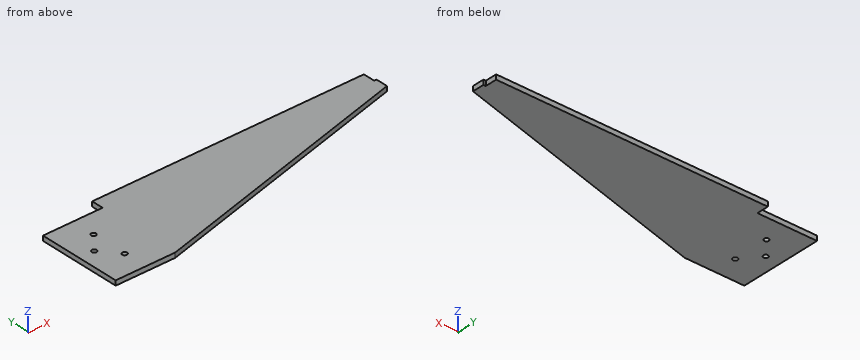
```python
from build123d import *

# Parameters (mm, degrees)
BOSS_EXTRUDE1_DEPTH = 4
BOSS_EXTRUDE2_DEPTH = 4
CUT_EXTRUDE1_REACH  = 6
SKETCH3_R           = 2


with BuildPart() as part:
    # Sketch1 → Boss-Extrude1 (new body)
    with BuildSketch(Plane.XY):
        Polygon((128, 30.092990436), (128, 40.092990436), (-100, 40.092990436), (-100, 20.092990436), (-130, 20.092990436), (-130, -39.907009564), (-100, -39.907009564), (130, 20.092990436), (130, 30.092990436), align=None)
    extrude(amount=BOSS_EXTRUDE1_DEPTH)

    # Sketch2 → Boss-Extrude2 (add)
    with BuildSketch(Plane.XY.offset(4)):
        Polygon((-100, 30.092990436), (-150, 30.092990436), (-150, -39.907009564), (-130, -39.907009564), (-130, 20.092990436), (-100, 20.092990436), align=None)
    extrude(amount=-BOSS_EXTRUDE2_DEPTH)

    # Sketch3 → Cut-Extrude1 (cut, up to next)
    with BuildSketch(Plane.XY.offset(4), mode=Mode.PRIVATE) as cut_extrude1_sk1:
        with Locations((-125, 10.092990436)):
            Circle(SKETCH3_R)
    cut_extrude1_tool1 = extrude(cut_extrude1_sk1.sketch, amount=-CUT_EXTRUDE1_REACH, mode=Mode.PRIVATE) & part.part
    add(cut_extrude1_tool1.solids().sort_by_distance((-125, 10.09299, 4))[0], mode=Mode.SUBTRACT)
    # Sketch3 → Cut-Extrude1 (cut, up to next)
    with BuildSketch(Plane.XY.offset(4), mode=Mode.PRIVATE) as cut_extrude1_sk2:
        with Locations((-125, -19.907009564)):
            Circle(SKETCH3_R)
    cut_extrude1_tool2 = extrude(cut_extrude1_sk2.sketch, amount=-CUT_EXTRUDE1_REACH, mode=Mode.PRIVATE) & part.part
    add(cut_extrude1_tool2.solids().sort_by_distance((-125, -19.90701, 4))[0], mode=Mode.SUBTRACT)
    # Sketch3 → Cut-Extrude1 (cut, up to next)
    with BuildSketch(Plane.XY.offset(4), mode=Mode.PRIVATE) as cut_extrude1_sk3:
        with Locations((-137.5, -4.907009564)):
            Circle(SKETCH3_R)
    cut_extrude1_tool3 = extrude(cut_extrude1_sk3.sketch, amount=-CUT_EXTRUDE1_REACH, mode=Mode.PRIVATE) & part.part
    add(cut_extrude1_tool3.solids().sort_by_distance((-137.5, -4.90701, 4))[0], mode=Mode.SUBTRACT)


solid = part.part
```
Geometry: final body of the model. Coordinates: model frame, mm. Give positions to 0.01 mm unless a question says otherwise; leave off trailing zeros. Write each loop counter-clockwise with the first axis right and the second up, starting at its lowest first coordinate (ties: lowest second). Pieces come first, ordered by that corner, then holes.
1. Section query B-B, the plane x = -57.5. Return loops of the section in (y, z).
2. Section query C-C, the plane y = -35. Return loops of the section in (x, z), then the cut area to 3 significant figures.
3. Pin query (flat end, axial travel): P1, Ø1.6, axis at x = 129, z = 2, coming from the +Y side; P2, Ø2, axis at x = 58, z = 2, coming from the -Y side; P3, Ø1, axis at x = 40.5, z = 0.5, coming from the -Y side. Return the tip coordinate at first contact, or that it passes through.
4. Section query A-A, the plane z = 2.95. Return loops of the section in (x, y), then the cut area to 3 significant figures.
5. Line query: probe 1 along Y at (x, z) = (-125, 1.15); probe 2 along Y at (x, z) = (-137.5, 2.6); probe 3 along X at (y, z) = (32, 2.35). Output: solid intervals per line, ascending.
Computed:
1. outline: (-28.82, 0) - (40.09, 0) - (40.09, 4) - (-28.82, 4) - close
2. outline: (-150, 0) - (-81.19, 0) - (-81.19, 4) - (-150, 4) - close
2. area: 275 mm2
3. P1: stops at y = 30.09
3. P2: stops at y = 1.05
3. P3: stops at y = -3.39
4. outline: (-150, -39.91) - (-100, -39.91) - (130, 20.09) - (130, 30.09) - (128, 30.09) - (128, 40.09) - (-100, 40.09) - (-100, 30.09) - (-150, 30.09) - close; hole circle Ø4 at (-137.5, -4.91); hole circle Ø4 at (-125, -19.91); hole circle Ø4 at (-125, 10.09)
4. area: 14,900 mm2
5. probe 1: y = -39.91 to -21.91, -17.91 to 8.09, 12.09 to 30.09
5. probe 2: y = -39.91 to -6.91, -2.91 to 30.09
5. probe 3: x = -100 to 128
